Geometry check sheet. Reference: the model listing, model coordinates, mm. Face numbers are marked on the shaded views. Coordinates: 2 decimals unless noted, no trailing zeros. Order: outer loops, then holes, each group sorted by start corner. A loop starts at its lowest first (then second) coordinate and runs counter-clockwise, first axis right, second up. Notation, with made-up numbers: (56.25, -15) -> (88.25, -15) arc R4 cw to (88.25, -9) -> close; hole circle Ø1 at (2.5, 6.25). An arc over 180 degrees is marked (long way). Answer in a Markdown table with one row per item. Add a question column.
```python
from build123d import *

# Parameters (mm, degrees)
SKETCH3_W                    = 130
SKETCH3_H                    = 95
BASE_FLANGE1_DEPTH           = 6.35
EDGE_FLANGE1_STRIP_W         = 26.8732
EDGE_FLANGE1_STRIP_H         = 6.35
EDGE_FLANGE1_STRIP_CUT_DEPTH = 95
EDGE_FLANGE1_DEPTH           = 95
EDGE_FLANGE1_PROFILE_W       = 95
EDGE_FLANGE1_PROFILE_H       = 210.4009
EDGE_FLANGE1_PROFILE_R       = 7.9375
EDGE_FLANGE1_FLAT_DEPTH      = 6.35
FILLET1_R                    = 25


# Sheet-metal steps are written as plain solids
with BuildPart() as part:
    # Sketch3 → Base-Flange1 (new body)
    with BuildSketch(Plane(origin=(0, 0, 0), x_dir=(1, 0, 0), z_dir=(0, 1, 0))):
        Rectangle(SKETCH3_W, SKETCH3_H)
    extrude(amount=-BASE_FLANGE1_DEPTH)

    # Edge-Flange1 strip (across the edge) → Edge-Flange1 strip cut (cut)
    with BuildSketch(Plane(origin=(65, -6.35, -47.5), x_dir=(-1, 0, 0), z_dir=(0, 0, 1))):
        with Locations((-6.35, -3.175)):
            Rectangle(EDGE_FLANGE1_STRIP_W, EDGE_FLANGE1_STRIP_H)
    edge_flange1_strip_cut = extrude(amount=EDGE_FLANGE1_STRIP_CUT_DEPTH, mode=Mode.SUBTRACT)

    # Edge-Flange1 bend section (across the edge) → Edge-Flange1 (add)
    with BuildSketch(Plane(origin=(65, -6.35, -47.5), x_dir=(-1, 0, 0), z_dir=(0, 0, 1))):
        with BuildLine():
            Line((0, 0.7366), (6.35, 0.7366))
            ThreePointArc((6.35, 0.7366), (6.565745145, 0.215745145), (7.0866, 0))
            Line((7.0866, 0), (7.0866, -6.35))
            ThreePointArc((7.0866, -6.35), (2.075617084, -4.274382916), (0, 0.7366))
        make_face()
    edge_flange1 = extrude(amount=EDGE_FLANGE1_DEPTH)

    # Edge-Flange1 profile (on flange) → Edge-Flange1 flat (add)
    with BuildSketch(Plane(origin=(65, -6.35, 0), x_dir=(0, 0, -1), z_dir=(-1, 0, 0))):
        with Locations((0, 105.93705)):
            Rectangle(EDGE_FLANGE1_PROFILE_W, EDGE_FLANGE1_PROFILE_H)
        with Locations((0, 177.8)):
            Circle(EDGE_FLANGE1_PROFILE_R, mode=Mode.SUBTRACT)
    edge_flange1_flat = extrude(amount=EDGE_FLANGE1_FLAT_DEPTH)

    # Mirror1: Edge-Flange1 strip cut, Edge-Flange1, Edge-Flange1 flat across plane
    add(edge_flange1_strip_cut.mirror(Plane(origin=(0, 0, 0), x_dir=(0, 0, 1), z_dir=(1, 0, 0))), mode=Mode.SUBTRACT)
    add(edge_flange1.mirror(Plane(origin=(0, 0, 0), x_dir=(0, 0, 1), z_dir=(1, 0, 0))))
    add(edge_flange1_flat.mirror(Plane(origin=(0, 0, 0), x_dir=(0, 0, 1), z_dir=(1, 0, 0))))

    # Fillet1
    fillet1_edges = [part.edges().sort_by_distance(p)[0] for p in [
        (61.825, -217.4875, -47.5),
        (61.825, -217.4875, 47.5),
        (-61.825, -217.4875, 47.5),
        (-61.825, -217.4875, -47.5),
    ]]
    fillet(fillet1_edges, radius=FILLET1_R)


solid = part.part
```
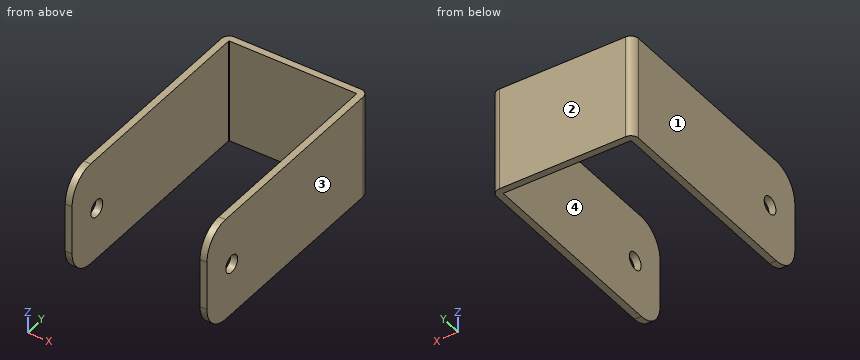
(1) Cross-section at A-A (y = -32). Enter the section's corners in (x, z), plus the area to 3 significant figures.
(2) Cross-section at B-B (z = 0). Enter the section's corners in (x, y).
(3) Scan lines: line 1 along X through (y, z) = (-135, 19); line 2 along Z through (x, y) = (60.75, -184.15); line 3 along Y through (x, z) = (-48, -4). Record each from-to range of solid material in increasing order.
(4) Cross-section at D-D (z = 16). Enter the section's corners in (x, y).
(5) Cross-section at C-C (y = -184.15). Enter the section's corners in (x, z), plus the area to 3 significant figures.
(6) Mould release check, pull along X, two halves, no side actions. Record for the marked faces 1, 2, 3 and 4: +X half, -X half, draft (parallel to the pull), parting line (faces both ways), or undercut.
(7) Go/stop test with flat-tipped pins: P1, Ø2, axis at x = 12.5, z = 9.5, coming from the -Y side; P2, Ø6, axis at x = 10.5, z = -2.5, coming from the +Y side. Record where each tip stops, or that it passes through.
Checks:
| question | item | result |
|---|---|---|
| 1 | outline | (-65, -47.5) -> (-58.65, -47.5) -> (-58.65, 47.5) -> (-65, 47.5) -> close; (58.65, -47.5) -> (65, -47.5) -> (65, 47.5) -> (58.65, 47.5) -> close |
| 1 | area | 1,210 mm² |
| 2 | outline | (-65, -217.49) -> (-58.65, -217.49) -> (-58.65, -192.09) -> (-65, -192.09) -> close; (-65, -176.21) -> (-58.65, -176.21) -> (-58.65, -7.09) arc R0.74 cw to (-57.91, -6.35) -> (57.91, -6.35) arc R0.74 cw to (58.65, -7.09) -> (58.65, -176.21) -> (65, -176.21) -> (65, -7.09) arc R7.09 ccw to (57.91, 0) -> (-57.91, 0) arc R7.09 ccw to (-65, -7.09) -> close; (58.65, -217.49) -> (65, -217.49) -> (65, -192.09) -> (58.65, -192.09) -> close |
| 3 | line 1 | -65 to -58.65, 58.65 to 65 |
| 3 | line 2 | -47.5 to -7.94, 7.94 to 47.5 |
| 3 | line 3 | -6.35 to 0 |
| 4 | outline | (-65, -217.49) -> (-58.65, -217.49) -> (-58.65, -7.09) arc R0.74 cw to (-57.91, -6.35) -> (57.91, -6.35) arc R0.74 cw to (58.65, -7.09) -> (58.65, -217.49) -> (65, -217.49) -> (65, -7.09) arc R7.09 ccw to (57.91, 0) -> (-57.91, 0) arc R7.09 ccw to (-65, -7.09) -> close |
| 5 | outline | (-65, -47.5) -> (-58.65, -47.5) -> (-58.65, -7.94) -> (-65, -7.94) -> close; (-65, 7.94) -> (-58.65, 7.94) -> (-58.65, 47.5) -> (-65, 47.5) -> close; (58.65, -47.5) -> (65, -47.5) -> (65, -7.94) -> (58.65, -7.94) -> close; (58.65, 7.94) -> (65, 7.94) -> (65, 47.5) -> (58.65, 47.5) -> close |
| 5 | area | 1,000 mm² |
| 6 | face 1 | -X half |
| 6 | face 2 | draft |
| 6 | face 3 | +X half |
| 6 | face 4 | undercut |
| 7 | P1 | y = -6.35 |
| 7 | P2 | y = 0 |
